CAD build for the part. Positions are in the model's coordinates, mm. A direction names the side the tool comes from. Coordinates: 2 decimals unless noted, no trailing zeros. Loops run counter-clockwise (first coordinate to the right, second up) from the corner with the lowest first, then second, coordinate; pieces in that order, holes last. Notation, with made-up numbers: (59, -9.5) - (111, -9.5) arc R16 cw to (111, 4.5) - close; hole circle Ø3 at (-33.5, 86.5). An arc over 180 degrees is marked (long way). Put each result on its own line as item: value.
```python
from build123d import *

# Parameters (mm, degrees)
SKETCH1_R           = 32.5
BOSS_EXTRUDE1_DEPTH = 2
SKETCH2_R           = 32.5
BOSS_EXTRUDE2_DEPTH = 13
CUT_EXTRUDE2_REACH  = 50.348
SKETCH3_R           = 5
CUT_EXTRUDE3_REACH  = 50.348
SKETCH5_R           = 1.3


with BuildPart() as part:
    # Sketch1 → Boss-Extrude1 (new body)
    with BuildSketch(Plane(origin=(0, 0, 0), x_dir=(1, 0, 0), z_dir=(0, 1, 0))):
        with Locations(Location((0, 0, 0), (0, 0, 270))):
            Circle(SKETCH1_R)
    extrude(amount=BOSS_EXTRUDE1_DEPTH)

    # Sketch2 → Boss-Extrude2 (add)
    with BuildSketch(Plane(origin=(0, 2, 0), x_dir=(1, 0, 0), z_dir=(0, 1, 0))):
        with Locations(Location((0, 0, 0), (0, 0, 270))):
            Circle(SKETCH2_R)
        with BuildLine():
            Line((2.6, -27.125679715), (2.6, -30))
            Line((2.6, -30), (-2.6, -30))
            Line((-2.6, -30), (-2.6, -27.125679715))
            ThreePointArc((-2.6, -27.125679715), (-19.268659787, -19.268659787), (-27.125679715, -2.6))
            Line((-27.125679715, -2.6), (-30, -2.6))
            Line((-30, -2.6), (-30, 2.6))
            Line((-30, 2.6), (-27.125679715, 2.6))
            ThreePointArc((-27.125679715, 2.6), (-19.268659787, 19.268659787), (-2.6, 27.125679715))
            Line((-2.6, 27.125679715), (-2.6, 30))
            Line((-2.6, 30), (2.6, 30))
            Line((2.6, 30), (2.6, 27.125679715))
            ThreePointArc((2.6, 27.125679715), (19.268659787, 19.268659787), (27.125679715, 2.6))
            Line((27.125679715, 2.6), (30, 2.6))
            Line((30, 2.6), (30, -2.6))
            Line((30, -2.6), (27.125679715, -2.6))
            ThreePointArc((27.125679715, -2.6), (19.268659787, -19.268659787), (2.6, -27.125679715))
        make_face(mode=Mode.SUBTRACT)
    extrude(amount=BOSS_EXTRUDE2_DEPTH)

    # Sketch3 → Cut-Extrude2 (cut, up to next)
    with BuildSketch(Plane.XZ, mode=Mode.PRIVATE) as cut_extrude2_sk1:
        with Locations(Location((0, 0, 0), (0, 0, 270))):
            Circle(SKETCH3_R)
    cut_extrude2_tool1 = extrude(cut_extrude2_sk1.sketch, amount=-CUT_EXTRUDE2_REACH, mode=Mode.PRIVATE) & part.part
    add(cut_extrude2_tool1.solids().sort_by_distance((0, 0, 0))[0], mode=Mode.SUBTRACT)

    # Sketch5 → Cut-Extrude3 (cut, up to next)
    with BuildSketch(Plane.XZ, mode=Mode.PRIVATE) as cut_extrude3_sk1:
        with Locations(Location((9, 5.5, 0), (0, 0, 270))):
            Circle(SKETCH5_R)
    cut_extrude3_tool1 = extrude(cut_extrude3_sk1.sketch, amount=-CUT_EXTRUDE3_REACH, mode=Mode.PRIVATE) & part.part
    # Sketch5 → Cut-Extrude3 (cut, up to next)
    with BuildSketch(Plane.XZ, mode=Mode.PRIVATE) as cut_extrude3_sk2:
        with Locations(Location((9, -5.5, 0), (0, 0, 270))):
            Circle(SKETCH5_R)
    cut_extrude3_tool2 = extrude(cut_extrude3_sk2.sketch, amount=-CUT_EXTRUDE3_REACH, mode=Mode.PRIVATE) & part.part
    # Sketch5 → Cut-Extrude3 (cut, up to next)
    with BuildSketch(Plane.XZ, mode=Mode.PRIVATE) as cut_extrude3_sk3:
        with Locations(Location((-9, -5.5, 0), (0, 0, 270))):
            Circle(SKETCH5_R)
    cut_extrude3_tool3 = extrude(cut_extrude3_sk3.sketch, amount=-CUT_EXTRUDE3_REACH, mode=Mode.PRIVATE) & part.part
    # Sketch5 → Cut-Extrude3 (cut, up to next)
    with BuildSketch(Plane.XZ, mode=Mode.PRIVATE) as cut_extrude3_sk4:
        with Locations(Location((-9, 5.5, 0), (0, 0, 270))):
            Circle(SKETCH5_R)
    cut_extrude3_tool4 = extrude(cut_extrude3_sk4.sketch, amount=-CUT_EXTRUDE3_REACH, mode=Mode.PRIVATE) & part.part
    add(cut_extrude3_tool1.solids().sort_by_distance((9, 0, 5.5))[0], mode=Mode.SUBTRACT)
    add(cut_extrude3_tool2.solids().sort_by_distance((9, 0, -5.5))[0], mode=Mode.SUBTRACT)
    add(cut_extrude3_tool3.solids().sort_by_distance((-9, 0, -5.5))[0], mode=Mode.SUBTRACT)
    add(cut_extrude3_tool4.solids().sort_by_distance((-9, 0, 5.5))[0], mode=Mode.SUBTRACT)


solid = part.part
```
Q1. Slice it at A-A, the plane x = 0. Give the cut face in (y, z).
Determined:
outline: (0, -32.5) - (15, -32.5) - (15, -30) - (2, -30) - (2, -5) - (0, -5) - close; (0, 5) - (2, 5) - (2, 30) - (15, 30) - (15, 32.5) - (0, 32.5) - close
Q2. Slice it at C-C, the plane z = 0. Give the cut face in (x, y), then the cut area to 3 significant figures.
Determined:
outline: (-32.5, 0) - (-5, 0) - (-5, 2) - (-30, 2) - (-30, 15) - (-32.5, 15) - close; (5, 0) - (32.5, 0) - (32.5, 15) - (30, 15) - (30, 2) - (5, 2) - close
area: 175 mm2
Q3. Slice it at D-D, the plane x = 9. Give the cut face in (y, z), then the cut area to 3 significant figures.
Determined:
outline: (0, -31.23) - (15, -31.23) - (15, -25.72) - (2, -25.72) - (2, -6.8) - (0, -6.8) - close; (0, -4.2) - (2, -4.2) - (2, 4.2) - (0, 4.2) - close; (0, 6.8) - (2, 6.8) - (2, 25.72) - (15, 25.72) - (15, 31.23) - (0, 31.23) - close
area: 258 mm2
Q4. Slice it at B-B, the plane y = 12.25. Give the cut face in (x, z).
Determined:
outline: circle Ø65 at (0, 0); hole (-30, -2.6) - (-27.13, -2.6) arc R27.25 ccw to (-2.6, -27.13) - (-2.6, -30) - (2.6, -30) - (2.6, -27.13) arc R27.25 ccw to (27.13, -2.6) - (30, -2.6) - (30, 2.6) - (27.13, 2.6) arc R27.25 ccw to (2.6, 27.13) - (2.6, 30) - (-2.6, 30) - (-2.6, 27.13) arc R27.25 ccw to (-27.13, 2.6) - (-30, 2.6) - close
Q5. Wall check: L1, parallel to X at y = 1, z = -5.5; L2, parallel to X at y = 0.95, z = 0; L3, parallel to Z at x = 17, y = 3.75. Give the ranges that are in metal, low to high. Write a range as from..to.
Determined:
L1: -32.03..-10.3, -7.7..7.7, 10.3..32.03
L2: -32.5..-5, 5..32.5
L3: -27.7..-21.3, 21.3..27.7
Q6. Pin check, flat tips, straight feed: pin 1 Ø1.5 at (x, y) = (22, 10) entering from +Z; pin 2 Ø3 at (y, z) = (11.5, 28.5) entering from -X; pin 3 Ø5 at (x, y) = (19, 5.5) entering from -Z; pin 4 Ø1.6 at (x, z) = (-9, -5.5) entering from -Y. Stop position of each tip, or through.
Determined:
pin 1: z = 24.59
pin 2: x = -18.09
pin 3: z = -28
pin 4: through
Q7. Tool access for faces 3 (the flat face through (0, 8, -30)), 4 (the flat face through (27, 15, -7)): list every direction of +Z, -Z, +X, -X, +Y, -Y with a clear straight run to the whole face (end or side of a thin tool).
Determined:
face 3: +Y
face 4: +Z, -Z, +X, -X, +Y
Q8. Mould opens along X. For faces 1 (the flat face through (0, 0, 7)), 2 (the cylindrical face through (9.39, 0.99, 4.26)) say: +X half, -X half, draft (parallel to the pull), parting line (faces both ways), or undercut.
Determined:
face 1: draft
face 2: undercut
